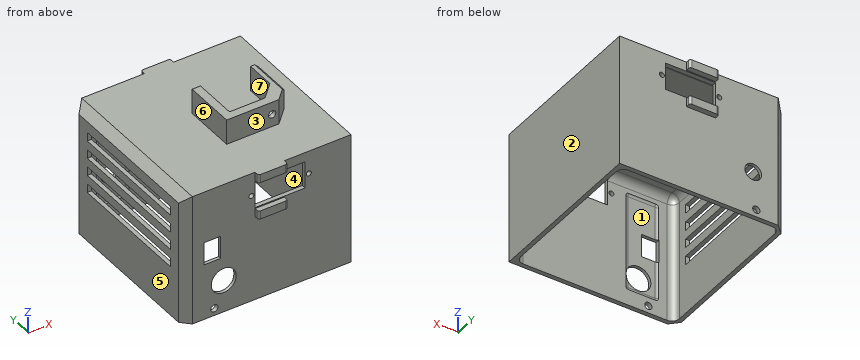
from build123d import *

# Parameters (mm, degrees)
CYLINDER070_R           = 1.75
CYLINDER070_DEPTH       = 20
CYLINDER070_PITCH_ANGLE = -90
PRISM_DEPTH             = 10
PRISM_PITCH_ANGLE       = -90
CYLINDER069_R           = 1
CYLINDER069_DEPTH       = 20
CYLINDER069_PITCH_ANGLE = -90
CYLINDER068_R           = 1
CYLINDER068_DEPTH       = 20
CYLINDER068_PITCH_ANGLE = -90
PAD008_DEPTH            = 13
CHAMFER106_SIZE         = 7
CUT094_PLACEMENT_ANGLE  = -90
CHAMFER107_SIZE         = 2
BOX053_W                = 7
BOX053_H                = 17
BOX053_DEPTH            = 15
BOX053_PLACEMENT_ANGLE  = -90
SKETCH011_R             = 1.2
SKETCH011_W             = 24
SKETCH011_H             = 13
PAD006_DEPTH            = 140
SKETCH009_W             = 60
SKETCH009_H             = 4.25
PAD004_DEPTH            = 45
BOX051_W                = 14
BOX051_H                = 3
BOX051_DEPTH            = 4
BOX050_W                = 14
BOX050_H                = 3
BOX050_DEPTH            = 4
BOX049_W                = 14
BOX049_H                = 3
BOX049_DEPTH            = 4
BOX020_W                = 8
BOX020_H                = 24
BOX020_DEPTH            = 11
CYLINDER026_R           = 4
CYLINDER026_DEPTH       = 31
CYLINDER026_ROLL_ANGLE  = 90
CYLINDER016_R           = 6
CYLINDER016_DEPTH       = 31
CYLINDER016_ROLL_ANGLE  = 90
CYLINDER015_R           = 1.75
CYLINDER015_DEPTH       = 31
CYLINDER015_ROLL_ANGLE  = 90
CYLINDER014_R           = 1.75
CYLINDER014_DEPTH       = 31
CYLINDER014_ROLL_ANGLE  = 90
BOX047_W                = 17
BOX047_H                = 77
BOX047_DEPTH            = 49
FILLET018014_R          = 2
BOX019_W                = 76
BOX019_H                = 76
BOX019_DEPTH            = 66
FILLET006_R             = 3.5
BOX048_W                = 80
BOX048_H                = 80
BOX048_DEPTH            = 63
CHAMFER103_SIZE         = 4
BOX052_W                = 14
BOX052_H                = 3
BOX052_DEPTH            = 4
FILLET018013002_R       = 1


with BuildPart() as cylinder070:
    # Cylinder070 → Cylinder070 (new body)
    with BuildSketch(Plane.XY):
        Circle(CYLINDER070_R)
    extrude(amount=CYLINDER070_DEPTH)


with BuildPart() as cylinder070_1:
    # Cylinder070 pitch: moved
    add(cylinder070.part.rotate(Axis((0, 0, 0), (0, 1, 0)), CYLINDER070_PITCH_ANGLE))


with BuildPart() as cylinder070_2:
    # Cylinder070 placement: moved
    add(cylinder070_1.part.moved(Location((-7, 12.8, 202))))


with BuildPart() as fusion053:
    # Prism → Prism (new body)
    with BuildSketch(Plane.XY):
        Polygon((3.3, 0), (1.65, 2.857884), (-1.65, 2.857884), (-3.3, 0), (-1.65, -2.857884), (1.65, -2.857884), align=None)
    extrude(amount=PRISM_DEPTH)


with BuildPart() as fusion053_1:
    # Prism pitch: moved
    add(fusion053.part.rotate(Axis((0, 0, 0), (0, 1, 0)), PRISM_PITCH_ANGLE))


with BuildPart() as fusion053_2:
    # Prism placement: moved
    add(fusion053_1.part.moved(Location((-16, 12.8, 202))))

    # Fusion053: union Cylinder070
    add(cylinder070_2.part)


with BuildPart() as cylinder095:
    # Cylinder069 → Cylinder069 (new body)
    with BuildSketch(Plane.XY):
        Circle(CYLINDER069_R)
    extrude(amount=CYLINDER069_DEPTH)


with BuildPart() as cylinder095_1:
    # Cylinder069 pitch: moved
    add(cylinder095.part.rotate(Axis((0, 0, 0), (0, 1, 0)), CYLINDER069_PITCH_ANGLE))


with BuildPart() as cylinder095_2:
    # Cylinder069 placement: moved
    add(cylinder095_1.part.moved(Location((-33, 21, 202))))


with BuildPart() as fusion052:
    # Cylinder068 → Cylinder068 (new body)
    with BuildSketch(Plane.XY):
        Circle(CYLINDER068_R)
    extrude(amount=CYLINDER068_DEPTH)


with BuildPart() as fusion052_1:
    # Cylinder068 pitch: moved
    add(fusion052.part.rotate(Axis((0, 0, 0), (0, 1, 0)), CYLINDER068_PITCH_ANGLE))


with BuildPart() as fusion052_2:
    # Cylinder068 placement: moved
    add(fusion052_1.part.moved(Location((-33, -7, 202))))

    # Fusion052: union Cylinder095
    add(cylinder095_2.part)


with BuildPart() as fusion052_3:
    # Fusion052 placement: moved
    add(fusion052_2.part.moved(Location((5, 0, 0))))


with BuildPart() as chamfer107:
    # Sketch013 → Pad008 (new body)
    with BuildSketch(Plane.XY.offset(195)):
        Polygon((-39, 19), (-39, 23), (-14, 23), (-14, -9), (-39, -9), (-39, -5), (-18, -5), (-18, 19), align=None)
    extrude(amount=PAD008_DEPTH)

    # Chamfer106
    chamfer106_edges = [chamfer107.edges().sort_by_distance(p)[0] for p in [
        (-14, 23, 201.5),
        (-18, 19, 201.5),
    ]]
    chamfer(chamfer106_edges, length=CHAMFER106_SIZE)

    # Cut093: cut Fusion052
    add(fusion052_3.part, mode=Mode.SUBTRACT)

    # Cut094: cut Fusion053
    add(fusion053_2.part, mode=Mode.SUBTRACT)


with BuildPart() as chamfer107_1:
    # Cut094 placement: moved
    add(chamfer107.part.moved(Location((34, 4, -65))).rotate(Axis((34, 4, -65), (0, 0, 1)), CUT094_PLACEMENT_ANGLE))

    # Chamfer107
    chamfer107_edges = [chamfer107_1.edges().sort_by_distance(p)[0] for p in [
        (57, 34, 143),
    ]]
    chamfer(chamfer107_edges, length=CHAMFER107_SIZE)


with BuildPart() as chamfer107_2:
    # Chamfer107 placement: moved
    add(chamfer107_1.part.moved(Location((-13, 0, 0))))


with BuildPart() as cube077:
    # Box053 → Box053 (new body)
    with BuildSketch(Plane.XY):
        with Locations((3.5, 8.5)):
            Rectangle(BOX053_W, BOX053_H)
    extrude(amount=BOX053_DEPTH)


with BuildPart() as cube077_1:
    # Box053 placement: moved
    add(cube077.part.moved(Location((16, 29, 120))).rotate(Axis((16, 29, 120), (0, 0, 1)), BOX053_PLACEMENT_ANGLE))


with BuildPart() as pad006:
    # Sketch011 → Pad006 (new body)
    with BuildSketch(Plane(origin=(-0.25, -35, 0), x_dir=(1, 0, 0), z_dir=(0, -1, 0))):
        with Locations((37, 120)):
            Circle(SKETCH011_R)
        with Locations((9.5, 120)):
            Circle(SKETCH011_R)
        with Locations((23.25, 120)):
            Rectangle(SKETCH011_W, SKETCH011_H)
    extrude(amount=-PAD006_DEPTH)


with BuildPart() as fusion051:
    # Sketch009 → Pad004 (new body)
    with BuildSketch(Plane(origin=(-40, 0, 0), x_dir=(0, -1, 0), z_dir=(-1, 0, 0))):
        with Locations((-36, 119.625)):
            Rectangle(SKETCH009_W, SKETCH009_H)
        with Locations((-36, 111.125)):
            Rectangle(SKETCH009_W, SKETCH009_H)
        with Locations((-36, 102.625)):
            Rectangle(SKETCH009_W, SKETCH009_H)
        with Locations((-36, 94.125)):
            Rectangle(SKETCH009_W, SKETCH009_H)
    extrude(amount=-PAD004_DEPTH)

    # Fusion051: union Pad006
    add(pad006.part)


with BuildPart() as cubo002:
    # Box051 → Box051 (new body)
    with BuildSketch(Plane(origin=(11, 75.5, 127), x_dir=(1, 0, 0), z_dir=(0, 0, 1))):
        with Locations((7, 1.5)):
            Rectangle(BOX051_W, BOX051_H)
    extrude(amount=BOX051_DEPTH)


with BuildPart() as cubo001:
    # Box050 → Box050 (new body)
    with BuildSketch(Plane(origin=(11, -6.5, 127), x_dir=(1, 0, 0), z_dir=(0, 0, 1))):
        with Locations((7, 1.5)):
            Rectangle(BOX050_W, BOX050_H)
    extrude(amount=BOX050_DEPTH)


with BuildPart() as cubo:
    # Box049 → Box049 (new body)
    with BuildSketch(Plane(origin=(11, -6.5, 109), x_dir=(1, 0, 0), z_dir=(0, 0, 1))):
        with Locations((7, 1.5)):
            Rectangle(BOX049_W, BOX049_H)
    extrude(amount=BOX049_DEPTH)


with BuildPart() as cube020:
    # Box020 → Box020 (new body)
    with BuildSketch(Plane(origin=(-13.5, -13, 95), x_dir=(1, 0, 0), z_dir=(0, 0, 1))):
        with Locations((4, 12)):
            Rectangle(BOX020_W, BOX020_H)
    extrude(amount=BOX020_DEPTH)


with BuildPart() as cylinder029:
    # Cylinder026 → Cylinder026 (new body)
    with BuildSketch(Plane.XY):
        Circle(CYLINDER026_R)
    extrude(amount=CYLINDER026_DEPTH)


with BuildPart() as cylinder029_1:
    # Cylinder026 roll: moved
    add(cylinder029.part.rotate(Axis((0, 0, 0), (1, 0, 0)), CYLINDER026_ROLL_ANGLE))


with BuildPart() as cylinder029_2:
    # Cylinder026 placement: moved
    add(cylinder029_1.part.moved(Location((-7, 80, 89.6))))


with BuildPart() as cylinder004:
    # Cylinder016 → Cylinder016 (new body)
    with BuildSketch(Plane.XY):
        Circle(CYLINDER016_R)
    extrude(amount=CYLINDER016_DEPTH)


with BuildPart() as cylinder004_1:
    # Cylinder016 roll: moved
    add(cylinder004.part.rotate(Axis((0, 0, 0), (1, 0, 0)), CYLINDER016_ROLL_ANGLE))


with BuildPart() as cylinder004_2:
    # Cylinder016 placement: moved
    add(cylinder004_1.part.moved(Location((-4, 11, 83.5))))


with BuildPart() as cylinder003:
    # Cylinder015 → Cylinder015 (new body)
    with BuildSketch(Plane.XY):
        Circle(CYLINDER015_R)
    extrude(amount=CYLINDER015_DEPTH)


with BuildPart() as cylinder003_1:
    # Cylinder015 roll: moved
    add(cylinder003.part.rotate(Axis((0, 0, 0), (1, 0, 0)), CYLINDER015_ROLL_ANGLE))


with BuildPart() as cylinder003_2:
    # Cylinder015 placement: moved
    add(cylinder003_1.part.moved(Location((-8.5, 80, 71.5))))


with BuildPart() as cylinder002:
    # Cylinder014 → Cylinder014 (new body)
    with BuildSketch(Plane.XY):
        Circle(CYLINDER014_R)
    extrude(amount=CYLINDER014_DEPTH)


with BuildPart() as cylinder002_1:
    # Cylinder014 roll: moved
    add(cylinder002.part.rotate(Axis((0, 0, 0), (1, 0, 0)), CYLINDER014_ROLL_ANGLE))


with BuildPart() as cylinder002_2:
    # Cylinder014 placement: moved
    add(cylinder002_1.part.moved(Location((-8.5, 11, 71.5))))


with BuildPart() as fusion044:
    # Box047 → Box047 (new body)
    with BuildSketch(Plane(origin=(-14, -2.5, 75), x_dir=(1, 0, 0), z_dir=(0, 0, 1))):
        with Locations((8.5, 38.5)):
            Rectangle(BOX047_W, BOX047_H)
    extrude(amount=BOX047_DEPTH)

    # Fillet018014
    fillet018014_edges = [fusion044.edges().sort_by_distance(p)[0] for p in [
        (-14, -2.5, 99.5),
        (-14, 36, 124),
        (-14, 74.5, 99.5),
        (-14, 36, 75),
        (3, -2.5, 99.5),
        (3, 36, 124),
        (3, 74.5, 99.5),
        (3, 36, 75),
        (-5.5, -2.5, 75),
        (-5.5, -2.5, 124),
        (-5.5, 74.5, 75),
        (-5.5, 74.5, 124),
    ]]
    fillet(fillet018014_edges, radius=FILLET018014_R)

    # Fusion044: union Cube020, Cylinder029, Cylinder004, Cylinder003, Cylinder002
    add(cube020.part)
    add(cylinder029_2.part)
    add(cylinder004_2.part)
    add(cylinder003_2.part)
    add(cylinder002_2.part)


with BuildPart() as fillet006:
    # Box019 → Box019 (new body)
    with BuildSketch(Plane(origin=(-21, -2, 87), x_dir=(1, 0, 0), z_dir=(0, 0, 1))):
        with Locations((38, 38)):
            Rectangle(BOX019_W, BOX019_H)
    extrude(amount=BOX019_DEPTH)

    # Fillet006
    fillet006_edges = [fillet006.edges().sort_by_distance(p)[0] for p in [
        (-21, -2, 120),
        (-21, 36, 153),
        (-21, 74, 120),
        (55, -2, 120),
        (55, 36, 153),
        (55, 74, 120),
        (17, -2, 153),
        (17, 74, 153),
    ]]
    fillet(fillet006_edges, radius=FILLET006_R)


with BuildPart() as fillet006_1:
    # Fillet006 placement: moved
    add(fillet006.part.moved(Location((0, 0, -24))))


with BuildPart() as fusion049:
    # Box048 → Box048 (new body)
    with BuildSketch(Plane(origin=(-23, -4, 68), x_dir=(1, 0, 0), z_dir=(0, 0, 1))):
        with Locations((40, 40)):
            Rectangle(BOX048_W, BOX048_H)
    extrude(amount=BOX048_DEPTH)

    # Chamfer103
    chamfer103_edges = [fusion049.edges().sort_by_distance(p)[0] for p in [
        (-23, -4, 99.5),
        (-23, 36, 131),
        (-23, 76, 99.5),
    ]]
    chamfer(chamfer103_edges, length=CHAMFER103_SIZE)

    # Cut081: cut Fillet006
    add(fillet006_1.part, mode=Mode.SUBTRACT)

    # Cut082: cut Fusion044
    add(fusion044.part, mode=Mode.SUBTRACT)

    # Fusion048: union Cubo
    add(cubo.part)

    # Fusion049: union Cubo001
    add(cubo001.part)


with BuildPart() as obj1:
    # Box052 → Box052 (new body)
    with BuildSketch(Plane(origin=(11, 75.5, 109), x_dir=(1, 0, 0), z_dir=(0, 0, 1))):
        with Locations((7, 1.5)):
            Rectangle(BOX052_W, BOX052_H)
    extrude(amount=BOX052_DEPTH)

    # Fusion050: union Cubo002, Fusion049
    add(cubo002.part)
    add(fusion049.part)

    # Cut092: cut Fusion051
    add(fusion051.part, mode=Mode.SUBTRACT)

    # Fillet018013002
    fillet018013002_edges = [obj1.edges().sort_by_distance(p)[0] for p in [
        (25, 78.5, 111),
        (11, 78.5, 111),
        (11, 78.5, 129),
        (25, 78.5, 129),
        (11, -6.5, 129),
        (25, -6.5, 129),
        (11, -6.5, 111),
        (25, -6.5, 111),
    ]]
    fillet(fillet018013002_edges, radius=FILLET018013002_R)

    # Cut095: cut Cube077
    add(cube077_1.part, mode=Mode.SUBTRACT)

    # Fusion054: union Chamfer107
    add(chamfer107_2.part)


solid = obj1.part
Could you check a few things on this model? Use its own coordinates, in mm. Face numbers are marked on the shaded views. A direction names the side the tool comes from. Give positions to 0.01 mm unless a question says otherwise; leave off trailing zeros. Order: outer loops, then holes, each group sorted by start corner. A loop starts at its lowest first (then second) coordinate and runs counter-clockwise, first axis right, second up. Notation, with made-up numbers: (-12.75, 50) - (5.25, 50) arc R26 cw to (5.25, 67) - close; hole circle Ø4 at (61.25, 82). An arc over 180 degrees is marked (long way). Return JSON: item names as keys, results as strings. Group by question number.
Q1. Please list where these lines run through material, in increasing order: line 1 along X through (y, z) = (36.75, 137); line 2 along Y through (x, z) = (-12.5, 75.5); line 3 along Z through (x, y) = (-4, -3.2). Write a range as [from, to].
Q2. Suppose I cut it at D-D, the plane x = 9.25. Please give me the cut outline in (y, z).
Q3. Which directions (+Z, -Z, +X, -X, +Y, -Y) give clear straight access to the entire face, cutting with the end or side of a thin tool? Please do the marked faces 4, 5, 6 and 7.
Q4. Suppose I cut it at A-A, the plane x = 18. State how many separate pieces and enclosed holes the cut face has, and give its area (3 significant figures).
Q5. Thinking about a two-plate mould opening in Y: for the marked faces 1, 2 and 3, which applies, pulls with the +Y half, pulls with the -Y half, needs draft (parallel to the pull), parting line crosses it, or undercut?
Q6. Suppose I cut it at C-C, the plane z = 103.5. Please give me the cut outline in (x, y), and give its area (3 significant figures).
Q7. Will these pins go through, and if not, where does the flat tip stop? pin 1 Ø1.5 at (x, z) = (-12.5, 128.5) entering from -Y; pin 2 Ø1.6 at (y, z) = (-5, 111.5) entering from +X; pin 3 Ø5.5 at (x, z) = (-8.5, 71.5) entering from +Y.
Q8. Suppose I cut it at B-B, the plane y = 15. Please give me the cut outline in (x, z), and give its area (3 significant figures).
Resolved:
{
 "1": {"line 1": "x = [12, 13], [15, 16], [40, 41], [43, 44]", "line 2": "y = [-4, -2], [74, 76]", "line 3": "z = [68, 77.5], [89.5, 131]"},
 "2": {"outline": "(-4, 68) - (-2, 68) - (-2, 118.8) - (-4, 118.8) - close; (-4, 121.2) - (-2, 121.2) - (-2, 125.5) arc R3.5 cw to (1.5, 129) - (70.5, 129) arc R3.5 cw to (74, 125.5) - (74, 121.2) - (76, 121.2) - (76, 131) - (-4, 131) - close; (74, 68) - (76, 68) - (76, 118.8) - (74, 118.8) - close"},
 "3": {"face 4": "-Z", "face 5": "+Z, -Z, -X, +Y, -Y", "face 6": "+Z, -X, +Y, -Y", "face 7": "+Z, +Y"},
 "4": {"separate pieces": "4", "enclosed holes": "0", "area": "431 mm2"},
 "5": {"face 1": "undercut", "face 2": "needs draft", "face 3": "pulls with the -Y half"},
 "6": {"outline": "(-23, 0) - (-19, -4) - (-13.5, -4) - (-13.5, -2) - (-17.5, -2) arc R3.5 cw to (-21, 1.5) - (-21, 6) - (-23, 6) - close; (-23, 66) - (-21, 66) - (-21, 70.5) arc R3.5 cw to (-17.5, 74) - (-13.32, 74) arc R2 cw to (-12, 74.5) - (1, 74.5) arc R2 cw to (2.32, 74) - (51.5, 74) arc R3.5 cw to (55, 70.5) - (55, 1.5) arc R3.5 cw to (51.5, -2) - (2.32, -2) arc R2 cw to (1, -2.5) - (-5.5, -2.5) - (-5.5, -4) - (57, -4) - (57, 76) - (-19, 76) - (-23, 72) - close", "area": "471 mm2"},
 "7": {"pin 1": "stops at y = -4", "pin 2": "stops at x = 25", "pin 3": "stops at y = 76"},
 "8": {"outline": "(-23, 68) - (-21, 68) - (-21, 92) - (-23, 92) - close; (-23, 96.25) - (-21, 96.25) - (-21, 100.5) - (-23, 100.5) - close; (-23, 104.75) - (-21, 104.75) - (-21, 109) - (-23, 109) - close; (-23, 113.25) - (-21, 113.25) - (-21, 117.5) - (-23, 117.5) - close; (-23, 121.75) - (-21, 121.75) - (-21, 125.5) arc R3.5 cw to (-17.5, 129) - (51.5, 129) arc R3.5 cw to (55, 125.5) - (55, 68) - (57, 68) - (57, 131) - (-19, 131) - (-23, 127) - close", "area": "367 mm2"}
}
